Read the model definition and answer for the solid it produces. Units are mm, in the model's axes. A direction names the side the tool comes from. Give positions to 0.01 mm unless a question says otherwise; leave off trailing zeros. Order: outer loops, then holes, each group sorted by start corner. A loop starts at its lowest first (then second) coordinate and runs counter-clockwise, first axis right, second up. Notation, with made-up numbers: (-8, 16) - (40, 16) arc R23 cw to (40, 50) - close; hole circle Ø10 at (21.5, 35.25). An arc over 180 degrees is marked (long way). One line per item, written item: value. Start each with the question number.
```python
from build123d import *

# Parameters (mm, degrees)
SALIENTE_EXTRUIR1_DEPTH = 6
CROQUIS18_R             = 3.75
CORTAR_EXTRUIR2_DEPTH   = 100.239609028
CORTAR_EXTRUIR3_DEPTH   = 101.709979645
CROQUIS21_R             = 7
CROQUIS21_R_2           = 3.75
SALIENTE_EXTRUIR3_DEPTH = 4


with BuildPart() as part:
    # Croquis14 → Saliente-Extruir1 (new body)
    with BuildSketch(Plane(origin=(0, 0, 0), x_dir=(1, 0, 0), z_dir=(0, 1, 0))):
        with BuildLine():
            Line((0, 7), (-72.95836944, 7))
            ThreePointArc((-72.95836944, 7), (-76.785203763, 7.761204675), (-80.029437252, 9.928932188))
            Line((-80.029437252, 9.928932188), (-85.550252532, 15.449747468))
            ThreePointArc((-85.550252532, 15.449747468), (-95.206682203, 15.681422839), (-95.901175207, 6.047213638))
            ThreePointArc((-95.901175207, 6.047213638), (-93.729852734, 0), (-95.901175207, -6.047213638))
            ThreePointArc((-95.901175207, -6.047213638), (-95.206682203, -15.681422839), (-85.550252532, -15.449747468))
            Line((-85.550252532, -15.449747468), (-80.029437252, -9.928932188))
            ThreePointArc((-80.029437252, -9.928932188), (-76.785203763, -7.761204675), (-72.95836944, -7))
            Line((-72.95836944, -7), (0, -7))
            Line((0, -7), (0, 7))
        make_face()
    extrude(amount=SALIENTE_EXTRUIR1_DEPTH)

    # Croquis18 → Cortar-Extruir2 (cut, through all)
    with BuildSketch(Plane(origin=(0, 6, 0), x_dir=(1, 0, 0), z_dir=(0, 1, 0))):
        with Locations(Location((-90.5, -10.5, 0), (0, 0, 270))):
            Circle(CROQUIS18_R)
        with Locations(Location((-90.5, 10.5, 0), (0, 0, 90))):
            Circle(CROQUIS18_R)
    extrude(amount=-CORTAR_EXTRUIR2_DEPTH, mode=Mode.SUBTRACT)

    # Croquis16 → Cortar-Extruir3 (cut, through all)
    with BuildSketch(Plane.XY.offset(7)):
        with BuildLine():
            Line((-63.851106218, 2.999108248), (-63.400446165, 2.999108248))
            ThreePointArc((-63.400446165, 2.999108248), (-62.793533932, 3.736620744), (-62.576232944, 4.6667))
            ThreePointArc((-62.576232944, 4.6667), (-62.453168135, 5.374868347), (-62.098403746, 6))
            Line((-62.098403746, 6), (-65.15454931, 6))
            ThreePointArc((-65.15454931, 6), (-64.798764982, 5.375104926), (-64.67531944, 4.6667))
            ThreePointArc((-64.67531944, 4.6667), (-64.458018451, 3.736620744), (-63.851106218, 2.999108248))
        make_face()
        with BuildLine():
            Line((-59.662406218, 2.999108248), (-59.211746165, 2.999108248))
            ThreePointArc((-59.211746165, 2.999108248), (-58.604833932, 3.736620744), (-58.387532944, 4.6667))
            ThreePointArc((-58.387532944, 4.6667), (-58.264468135, 5.374868347), (-57.909703746, 6))
            Line((-57.909703746, 6), (-60.96584931, 6))
            ThreePointArc((-60.96584931, 6), (-60.610064982, 5.375104926), (-60.48661944, 4.6667))
            ThreePointArc((-60.48661944, 4.6667), (-60.269318451, 3.736620744), (-59.662406218, 2.999108248))
        make_face()
        with BuildLine():
            Line((-68.039806218, 2.999108248), (-67.589146165, 2.999108248))
            ThreePointArc((-67.589146165, 2.999108248), (-66.982233932, 3.736620744), (-66.764932944, 4.6667))
            ThreePointArc((-66.764932944, 4.6667), (-66.641868135, 5.374868347), (-66.287103746, 6))
            Line((-66.287103746, 6), (-69.34324931, 6))
            ThreePointArc((-69.34324931, 6), (-68.987464982, 5.375104926), (-68.86401944, 4.6667))
            ThreePointArc((-68.86401944, 4.6667), (-68.646718451, 3.736620744), (-68.039806218, 2.999108248))
        make_face()
        with BuildLine():
            Line((-55.473706218, 2.999108248), (-55.023046165, 2.999108248))
            ThreePointArc((-55.023046165, 2.999108248), (-54.416133932, 3.736620744), (-54.198832944, 4.6667))
            ThreePointArc((-54.198832944, 4.6667), (-54.075768135, 5.374868347), (-53.721003746, 6))
            Line((-53.721003746, 6), (-56.77714931, 6))
            ThreePointArc((-56.77714931, 6), (-56.421364982, 5.375104926), (-56.29791944, 4.6667))
            ThreePointArc((-56.29791944, 4.6667), (-56.080618451, 3.736620744), (-55.473706218, 2.999108248))
        make_face()
        with BuildLine():
            Line((-51.285006218, 2.999108248), (-50.834346165, 2.999108248))
            ThreePointArc((-50.834346165, 2.999108248), (-50.227433932, 3.736620744), (-50.010132944, 4.6667))
            ThreePointArc((-50.010132944, 4.6667), (-49.887068135, 5.374868347), (-49.532303746, 6))
            Line((-49.532303746, 6), (-52.58844931, 6))
            ThreePointArc((-52.58844931, 6), (-52.232664982, 5.375104926), (-52.10921944, 4.6667))
            ThreePointArc((-52.10921944, 4.6667), (-51.891918451, 3.736620744), (-51.285006218, 2.999108248))
        make_face()
        with BuildLine():
            Line((-47.096306218, 2.999108248), (-46.645646165, 2.999108248))
            ThreePointArc((-46.645646165, 2.999108248), (-46.038733932, 3.736620744), (-45.821432944, 4.6667))
            ThreePointArc((-45.821432944, 4.6667), (-45.698368135, 5.374868347), (-45.343603746, 6))
            Line((-45.343603746, 6), (-48.39974931, 6))
            ThreePointArc((-48.39974931, 6), (-48.043964982, 5.375104926), (-47.92051944, 4.6667))
            ThreePointArc((-47.92051944, 4.6667), (-47.703218451, 3.736620744), (-47.096306218, 2.999108248))
        make_face()
        with BuildLine():
            Line((-42.907606218, 2.999108248), (-42.456946165, 2.999108248))
            ThreePointArc((-42.456946165, 2.999108248), (-41.850033932, 3.736620744), (-41.632732944, 4.6667))
            ThreePointArc((-41.632732944, 4.6667), (-41.509668135, 5.374868347), (-41.154903746, 6))
            Line((-41.154903746, 6), (-44.21104931, 6))
            ThreePointArc((-44.21104931, 6), (-43.855264982, 5.375104926), (-43.73181944, 4.6667))
            ThreePointArc((-43.73181944, 4.6667), (-43.514518451, 3.736620744), (-42.907606218, 2.999108248))
        make_face()
        with BuildLine():
            Line((-38.718906218, 2.999108248), (-38.268246165, 2.999108248))
            ThreePointArc((-38.268246165, 2.999108248), (-37.661333932, 3.736620744), (-37.444032944, 4.6667))
            ThreePointArc((-37.444032944, 4.6667), (-37.320968135, 5.374868347), (-36.966203746, 6))
            Line((-36.966203746, 6), (-40.02234931, 6))
            ThreePointArc((-40.02234931, 6), (-39.666564982, 5.375104926), (-39.54311944, 4.6667))
            ThreePointArc((-39.54311944, 4.6667), (-39.325818451, 3.736620744), (-38.718906218, 2.999108248))
        make_face()
        with BuildLine():
            Line((-34.530206218, 2.999108248), (-34.079546165, 2.999108248))
            ThreePointArc((-34.079546165, 2.999108248), (-33.472633932, 3.736620744), (-33.255332944, 4.6667))
            ThreePointArc((-33.255332944, 4.6667), (-33.132268135, 5.374868347), (-32.777503746, 6))
            Line((-32.777503746, 6), (-35.83364931, 6))
            ThreePointArc((-35.83364931, 6), (-35.477864982, 5.375104926), (-35.35441944, 4.6667))
            ThreePointArc((-35.35441944, 4.6667), (-35.137118451, 3.736620744), (-34.530206218, 2.999108248))
        make_face()
        with BuildLine():
            Line((-30.341506218, 2.999108248), (-29.890846165, 2.999108248))
            ThreePointArc((-29.890846165, 2.999108248), (-29.283933932, 3.736620744), (-29.066632944, 4.6667))
            ThreePointArc((-29.066632944, 4.6667), (-28.943568135, 5.374868347), (-28.588803746, 6))
            Line((-28.588803746, 6), (-31.64494931, 6))
            ThreePointArc((-31.64494931, 6), (-31.289164982, 5.375104926), (-31.16571944, 4.6667))
            ThreePointArc((-31.16571944, 4.6667), (-30.948418451, 3.736620744), (-30.341506218, 2.999108248))
        make_face()
        with BuildLine():
            Line((-26.152806218, 2.999108248), (-25.702146165, 2.999108248))
            ThreePointArc((-25.702146165, 2.999108248), (-25.095233932, 3.736620744), (-24.877932944, 4.6667))
            ThreePointArc((-24.877932944, 4.6667), (-24.754868135, 5.374868347), (-24.400103746, 6))
            Line((-24.400103746, 6), (-27.45624931, 6))
            ThreePointArc((-27.45624931, 6), (-27.100464982, 5.375104926), (-26.97701944, 4.6667))
            ThreePointArc((-26.97701944, 4.6667), (-26.759718451, 3.736620744), (-26.152806218, 2.999108248))
        make_face()
        with BuildLine():
            Line((-21.964106218, 2.999108248), (-21.513446165, 2.999108248))
            ThreePointArc((-21.513446165, 2.999108248), (-20.906533932, 3.736620744), (-20.689232944, 4.6667))
            ThreePointArc((-20.689232944, 4.6667), (-20.566168135, 5.374868347), (-20.211403746, 6))
            Line((-20.211403746, 6), (-23.26754931, 6))
            ThreePointArc((-23.26754931, 6), (-22.911764982, 5.375104926), (-22.78831944, 4.6667))
            ThreePointArc((-22.78831944, 4.6667), (-22.571018451, 3.736620744), (-21.964106218, 2.999108248))
        make_face()
        with BuildLine():
            Line((-17.775406218, 2.999108248), (-17.324746165, 2.999108248))
            ThreePointArc((-17.324746165, 2.999108248), (-16.717833932, 3.736620744), (-16.500532944, 4.6667))
            ThreePointArc((-16.500532944, 4.6667), (-16.377468135, 5.374868347), (-16.022703746, 6))
            Line((-16.022703746, 6), (-19.07884931, 6))
            ThreePointArc((-19.07884931, 6), (-18.723064982, 5.375104926), (-18.59961944, 4.6667))
            ThreePointArc((-18.59961944, 4.6667), (-18.382318451, 3.736620744), (-17.775406218, 2.999108248))
        make_face()
        with BuildLine():
            Line((-13.586706218, 2.999108248), (-13.136046165, 2.999108248))
            ThreePointArc((-13.136046165, 2.999108248), (-12.529133932, 3.736620744), (-12.311832944, 4.6667))
            ThreePointArc((-12.311832944, 4.6667), (-12.188768135, 5.374868347), (-11.834003746, 6))
            Line((-11.834003746, 6), (-14.89014931, 6))
            ThreePointArc((-14.89014931, 6), (-14.534364982, 5.375104926), (-14.41091944, 4.6667))
            ThreePointArc((-14.41091944, 4.6667), (-14.193618451, 3.736620744), (-13.586706218, 2.999108248))
        make_face()
        with BuildLine():
            Line((-9.398006218, 2.999108248), (-8.947346165, 2.999108248))
            ThreePointArc((-8.947346165, 2.999108248), (-8.340433932, 3.736620744), (-8.123132944, 4.6667))
            ThreePointArc((-8.123132944, 4.6667), (-8.000068135, 5.374868347), (-7.645303746, 6))
            Line((-7.645303746, 6), (-10.70144931, 6))
            ThreePointArc((-10.70144931, 6), (-10.345664982, 5.375104926), (-10.22221944, 4.6667))
            ThreePointArc((-10.22221944, 4.6667), (-10.004918451, 3.736620744), (-9.398006218, 2.999108248))
        make_face()
        with BuildLine():
            Line((-5.209306218, 2.999108248), (-4.758646165, 2.999108248))
            ThreePointArc((-4.758646165, 2.999108248), (-4.151733932, 3.736620744), (-3.934432944, 4.6667))
            ThreePointArc((-3.934432944, 4.6667), (-3.811368135, 5.374868347), (-3.456603746, 6))
            Line((-3.456603746, 6), (-6.51274931, 6))
            ThreePointArc((-6.51274931, 6), (-6.156964982, 5.375104926), (-6.03351944, 4.6667))
            ThreePointArc((-6.03351944, 4.6667), (-5.816218451, 3.736620744), (-5.209306218, 2.999108248))
        make_face()
        with BuildLine():
            Line((-1.020606218, 2.999108248), (-0.569946165, 2.999108248))
            ThreePointArc((-0.569946165, 2.999108248), (0.036966068, 3.736620744), (0.254267056, 4.6667))
            ThreePointArc((0.254267056, 4.6667), (0.377331865, 5.374868347), (0.732096254, 6))
            Line((0.732096254, 6), (-2.32404931, 6))
            ThreePointArc((-2.32404931, 6), (-1.968264982, 5.375104926), (-1.84481944, 4.6667))
            ThreePointArc((-1.84481944, 4.6667), (-1.627518451, 3.736620744), (-1.020606218, 2.999108248))
        make_face()
    extrude(amount=-CORTAR_EXTRUIR3_DEPTH, mode=Mode.SUBTRACT)

    # Croquis21 → Saliente-Extruir3 (add)
    # profile 1 of 2: a face of its own
    with BuildSketch(Plane.XZ):
        with Locations(Location((-90.5, -10.5, 0), (0, 0, 270))):
            Circle(CROQUIS21_R)
        with Locations(Location((-90.5, -10.5, 0), (0, 0, 270))):
            Circle(CROQUIS21_R_2, mode=Mode.SUBTRACT)
    # profile 2 of 2: a face of its own
    with BuildSketch(Plane.XZ):
        with Locations(Location((-90.5, 10.5, 0), (0, 0, 219.502533363))):
            Circle(CROQUIS21_R)
        with Locations(Location((-90.5, 10.5, 0), (0, 0, 90))):
            Circle(CROQUIS21_R_2, mode=Mode.SUBTRACT)
    extrude(amount=SALIENTE_EXTRUIR3_DEPTH)


solid = part.part
```
1) Section C-C on z = 12.5 is taken. Write down the section's boundary in (x, y), plus the area to 3 significant figures.
2) Find the intervals of material crossed by probe 1 along Z at (x, y) = (-61.5, 3.75); probe 2 along Z at (x, y) = (-92.5, 4.5); probe 3 along Y at (x, z) = (-77.5, 6), in increasing order. Write a range as from..to.
3) Section A-A on y = 1 is taken. Write down the section's boundary in (x, z), plus the area to 3 significant figures.
4) The mould has two halves that part along X. Classify faces 3 (the flat face through (-82.8, 3, 12.7)), 4 (the flat face through (-36, 3, -7)), 5 (the cylindrical face through (-68.653, 3.749, 0.098)), 6 (the cylindrical face through (-10.01, 3.75, 0.1)): +X half, -X half, draft (parallel to the pull), parting line (faces both ways), or undercut.
5) Each of these flat-tipped pins is pushed along its axis until it touches: pin 1 (0.5 mm diameter, centred on x = -55, z = 3, fed in from +Y); pin 2 (6 mm diameter, centred on x = -16, y = 0.5, fed in from +Z); pin 3 (5 mm diameter, centred on x = -55.5, y = 4, fed in from -Z); pin 4 (2 mm diameter, centred on x = -35.5, y = -1.5, fed in from -Z). Where does it stop, or does it pass through?
6) Section D-D on y = -3 is taken. Write down the section's boundary in (x, z).
7) For faces 1 (the cylindrical face through (-43.52, 3.75, 0.1)), 2 (the cylindrical face through (-76.73, 2.96, -7.74)), determine the directions among +Z, -Z, +X, -X, +Y, -Y from which every point of the face is accessible in a straight line to the end or side of a thin tool.
8) Section B-B on x = -90.5 is taken. Write down the section's boundary in (y, z), plus the area to 3 significant figures.
Solved:
1. outline: (-97.21, -4) - (-93.67, -4) - (-93.67, 6) - (-97.21, 6) - close; (-87.33, -4) - (-83.79, -4) - (-83.79, 0) - (-82.6, 0) - (-82.6, 6) - (-87.33, 6) - close
1. area: 77.9 mm2
2. probe 1: z = -7..7
2. probe 2: z = -17.21..-13.67, -7.33..7.33, 13.67..17.21
2. probe 3: y = 0..6
3. outline: (-95.9, -6.05) arc R7 ccw to (-85.55, -15.45) - (-80.03, -9.93) arc R10 cw to (-72.96, -7) - (0, -7) - (0, 7) - (-72.96, 7) arc R10 cw to (-80.03, 9.93) - (-85.55, 15.45) arc R7 ccw to (-95.9, 6.05) arc R9.51 cw to start; hole circle Ø7.5 at (-90.5, -10.5); hole circle Ø7.5 at (-90.5, 10.5)
3. area: 1,530 mm2
4. face 3: +X half
4. face 4: draft
4. face 5: undercut
4. face 6: undercut
5. pin 1: stops at y = 3.25
5. pin 2: stops at z = 7
5. pin 3: stops at z = -7
5. pin 4: passes through
6. outline: circle Ø14 at (-90.5, -10.5); circle Ø14 at (-90.5, 10.5); hole circle Ø7.5 at (-90.5, -10.5); hole circle Ø7.5 at (-90.5, 10.5)
7. face 1: +Z, -Z, +Y
7. face 2: -Z, +X, +Y, -Y
8. outline: (-4, -17.5) - (6, -17.5) - (6, -14.25) - (-4, -14.25) - close; (-4, -6.75) - (6, -6.75) - (6, 6.75) - (-4, 6.75) - (-4, 3.5) - (0, 3.5) - (0, -3.5) - (-4, -3.5) - close; (-4, 14.25) - (6, 14.25) - (6, 17.5) - (-4, 17.5) - close
8. area: 172 mm2
